from build123d import *

# Parameters (mm, degrees)
SKETCH_1_W          = 68.2
SKETCH_1_H          = 17.95
EXTRUDE_1_DEPTH     = 3.5
SKETCH_21_W         = 68.2
SKETCH_21_H         = 3.5
EXTRUDE_4_DEPTH     = 28.25
SKETCH_24_R         = 2.85
CUT_EXTRUDE_2_DEPTH = 28.25
SKETCH_30_W         = 68.2
SKETCH_30_H         = 3.5
EXTRUDE_6_DEPTH     = 12
SKETCH_31_W         = 31.388626345
SKETCH_31_H         = 3.5
EXTRUDE_7_DEPTH     = 22
SKETCH_32_W         = 1.503469792
SKETCH_32_H         = 31.388626345
EXTRUDE_8_DEPTH     = 30


with BuildPart() as part:
    # 草圖1 → 1 (new body)
    with BuildSketch(Plane.XY):
        Rectangle(SKETCH_1_W, SKETCH_1_H)
    extrude(amount=EXTRUDE_1_DEPTH)

    # 草圖21 → 填料-伸長4 (add)
    with BuildSketch(Plane.XY.offset(3.5)):
        with Locations((0, 7.225)):
            Rectangle(SKETCH_21_W, SKETCH_21_H)
    extrude(amount=EXTRUDE_4_DEPTH)

    # 草圖24 → 除料-伸長2 (cut)
    with BuildSketch(Plane(origin=(0, 0, 0), x_dir=(-1, 0, 0), z_dir=(0, 0, -1))):
        with Locations((0, -3.070533486)):
            Circle(SKETCH_24_R)
    extrude(amount=-CUT_EXTRUDE_2_DEPTH, mode=Mode.SUBTRACT)

    # 草圖30 → 填料-伸長6 (add)
    with BuildSketch(Plane.XY.offset(31.75)):
        with Locations((0, 7.225)):
            Rectangle(SKETCH_30_W, SKETCH_30_H)
    extrude(amount=EXTRUDE_6_DEPTH)

    # 草圖31 → 填料-伸長7 (add)
    with BuildSketch(Plane.ZY.offset(34.1)):
        with Locations((28.055686828, 7.225)):
            Rectangle(SKETCH_31_W, SKETCH_31_H)
    extrude(amount=EXTRUDE_7_DEPTH)

    # 草圖32 → 填料-伸長8 (add)
    with BuildSketch(Plane(origin=(0, 8.975, 0), x_dir=(1, 0, 0), z_dir=(0, 1, 0))):
        with Locations((-55.348265104, -28.055686828)):
            Rectangle(SKETCH_32_W, SKETCH_32_H)
    extrude(amount=EXTRUDE_8_DEPTH)


solid = part.part
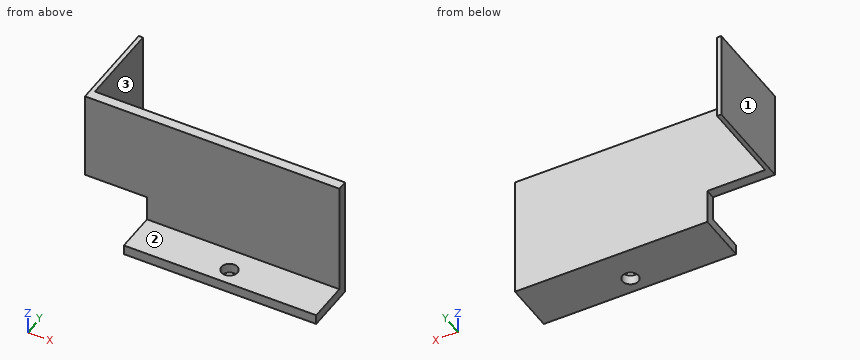
CAD build for the part. Positions are in the model's coordinates, mm. Face numbers are marked on the shaded views. A direction names the side the tool comes from. Round coordinates to 2 decimals unless told otherwise and drop trailing zeros. Loops run counter-clockwise (first coordinate to the right, second up) from the corner with the lowest first, then second, coordinate; pieces in that order, holes last. Notation, with made-up numbers: M -21.5,43.5 L 4.5,43.5 A30 cw 4.5,75.5 Z; hole C -34.75,38.5 d9. An arc over 180 degrees is marked long. One line per question, with ' | ' between items. Start each with the question number.
Item 1: Cut at A-A, the plane x = 0. Write the cut outline in (y, z) (3 decimals), plus the area to 3 significant figures.
Item 2: Which spindle directions (+Z, -Z, +X, -X, +Y, -Y) get a long thin tool onto all of the face, cutting with end or side? Do the marked faces 1, 2 and 3. Say none if no direction does.
Item 3: Cut at B-B, the plane y = 15. Write the cut outline in (x, z), plus the area to 3 significant figures.
Item 4: Pin check, flat tips, straight feed: pin 1 Ø12 at (x, z) = (9.5, 31.5) entering from -Y (3 decimals); pin 2 Ø17.5 at (x, y) = (-47.5, 14) entering from -Z; pin 3 Ø13 at (x, z) = (5.5, 25) entering from +Y (3 decimals). Stop position of each tip, or through.
Item 5: Wall check: line 1 (Y direction, x = 0, z = 2.65) (3 decimals); line 2 (X direction, y = 30.5, z = 28); line 3 (Y direction, x = 19.5, z = 39) (3 decimals). Give the ranges that are in metal, low to high.
Item 6: Cut at D-D, the plane x = -32. Write the cut outline in (y, z) (3 decimals).
Item 7: Cut at C-C, the plane z = 41. Write the cut outline in (x, y) (3 decimals).
Responses:
1) outline: M -8.975,0 L -5.921,0 L -5.921,3.5 L -8.975,3.5 Z; M -0.221,0 L 8.975,0 L 8.975,43.75 L 5.475,43.75 L 5.475,3.5 L -0.221,3.5 Z | area: 184 mm²
2) face 1: +Z, -Z, -X, +Y, -Y | face 2: +Z, +X, -X, -Y | face 3: +Z, -Z, +X, +Y
3) outline: M -56.1,12.36 L -54.6,12.36 L -54.6,43.75 L -56.1,43.75 Z | area: 47.2 mm²
4) pin 1: stops at y = 5.475 | pin 2: stops at z = 12.36 | pin 3: stops at y = 8.975
5) line 1: y = -8.975 to -5.921, -0.221 to 8.975 | line 2: x = -56.1 to -54.6 | line 3: y = 5.475 to 8.975
6) outline: M -8.975,0 L 8.975,0 L 8.975,43.75 L 5.475,43.75 L 5.475,3.5 L -8.975,3.5 Z
7) outline: M -56.1,5.475 L 34.1,5.475 L 34.1,8.975 L -54.597,8.975 L -54.597,38.975 L -56.1,38.975 Z
